Geometry check sheet. Reference: drawing and pictorial views, mm from the part's lowest x, y, z. A direction names the side the tool comes from. Coordinates: 2 decimals unless noted, no trailing zeros. Loops run counter-clockwise (first coordinate to the right, second up) from the corner with the lowest first, then second, coordinate; pieces in that order, holes last. Notation, with made-up numbers: (71.5, 36) -> (126.5, 36) arc R32 ccw to (126.5, 71) -> close; hole circle Ø1 at (38, 47.5). An arc over 180 degrees is marked (long way). Use CSV: the item, a comma, the result in double quotes.
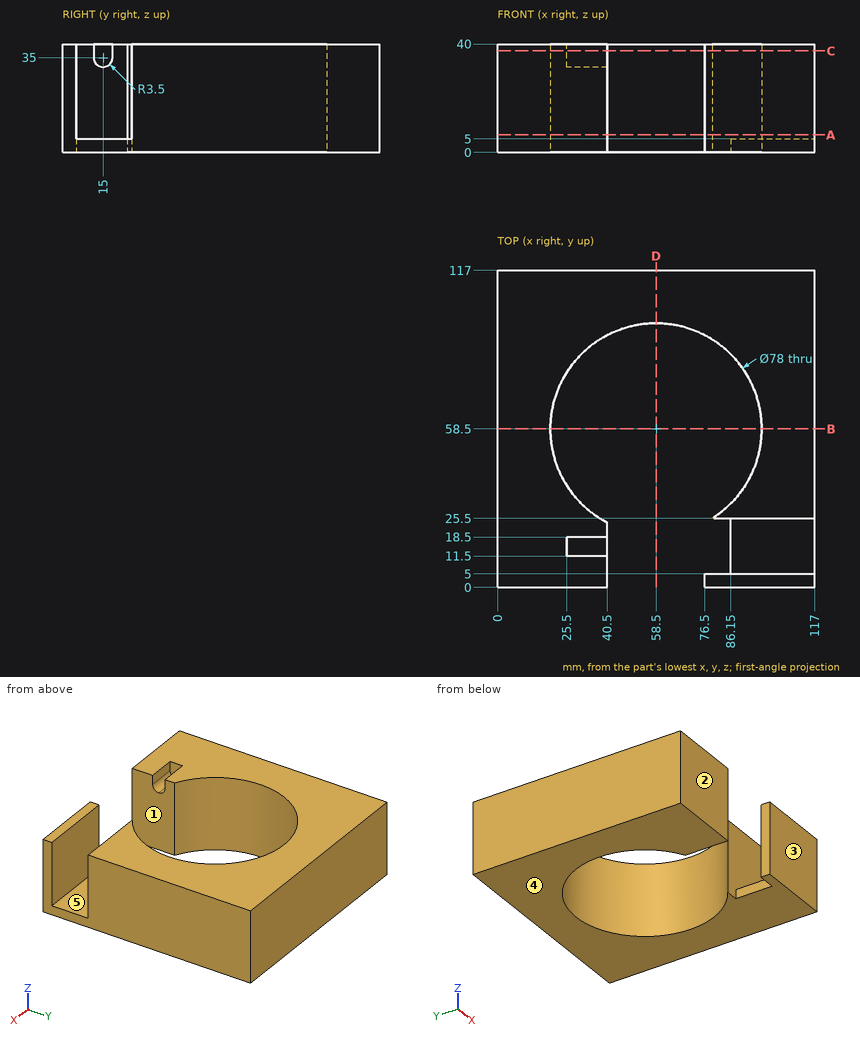
1) Cross-section at D-D on x = 58.5. Record the boundary of the cut face in (y, z), and give its area (3 significant figures).
Answer below:
outline,"(97.5, 0) -> (117, 0) -> (117, 40) -> (97.5, 40) -> close"
area,"780 mm²"
2) Cross-section at A-A on z = 6.5. Record the boundary of the cut face in (x, y), and give its area (3 significant figures).
Answer below:
outline,"(0, 0) -> (40.5, 0) -> (40.5, 23.9) arc R39 cw (long way) to (79.28, 25.5) -> (117, 25.5) -> (117, 117) -> (0, 117) -> close; (76.5, 0) -> (117, 0) -> (117, 5) -> (76.5, 5) -> close"
area,"7,330 mm²"
3) Cross-section at C-C on z = 37.5. Record the boundary of the cut face in (x, y), and give its area (3 significant figures).
Answer below:
outline,"(0, 0) -> (40.5, 0) -> (40.5, 11.5) -> (25.5, 11.5) -> (25.5, 18.5) -> (40.5, 18.5) -> (40.5, 23.9) arc R39 cw (long way) to (79.28, 25.5) -> (117, 25.5) -> (117, 117) -> (0, 117) -> close; (76.5, 0) -> (117, 0) -> (117, 5) -> (76.5, 5) -> close"
area,"7,220 mm²"
4) Access from +Z, -Z, +X, -X, +Y, -Y to the whole of each face (thin tool, end or side, straight path). Record for the marked faces 1 and 2.
Answer below:
face 1,"+Z, -Z, -Y"
face 2,"+Z, -Z, +X, -X, -Y"
5) Go/stop test with flat-tipped pins: pin 1 Ø7 at (y, z) = (12.5, 23.5) entering from +X; pin 2 Ø6 at (y, z) = (39.5, 21) entering from -X; pin 3 Ø1 at (x, z) = (54, 5) entering from -Y; pin 4 Ø6 at (x, y) = (97, 10.5) entering from +Z. Record where each tip stops, or that it passes through.
Answer below:
pin 1,"stops at x = 40.5"
pin 2,"stops at x = 0"
pin 3,"stops at y = 97.18"
pin 4,"stops at z = 5"
6) Thickness scan on line 1 along X through (y, z) = (58.5, 30.5); line 2 along Y through (x, z) = (93, 14.5); line 3 along X through (y, z) = (10.5, 23.5). Record the ranges inside material, lowest first. Write a range as from..to.
Answer below:
line 1,"x = 0..19.5, 97.5..117"
line 2,"y = 0..5, 25.5..40.31, 76.69..117"
line 3,"x = 0..40.5"
7) Cross-section at B-B on y = 58.5. Record the boundary of the cut face in (x, z), and give its area (3 significant figures).
Answer below:
outline,"(0, 0) -> (19.5, 0) -> (19.5, 40) -> (0, 40) -> close; (97.5, 0) -> (117, 0) -> (117, 40) -> (97.5, 40) -> close"
area,"1,560 mm²"
8) Draft check along Y on the marked faces 3, 4 and 5. Enter one of: released by +Y, released by -Y, zero draft, split by the parting line, or undercut.
Answer below:
face 3,"released by -Y"
face 4,"zero draft"
face 5,"undercut"
